Verification items for this drawing (mm, ordinates from the low corner). Give positions to 0.01 mm unless a question says otherwise; leave off trailing zeros. Order: outer loops, then holes, each group sorted by start corner. A loop starts at its lowest first (then second) coordinate and runs counter-clockwise, first axis right, second up. Notation, with made-up numbers: M 67,-14.75 L 82,-14.75 A33 ccw 82,16.25 Z; hole C -9,80.25 d8. An arc over 180 degrees is marked long. Answer as a JSON object with one key per item and string values.
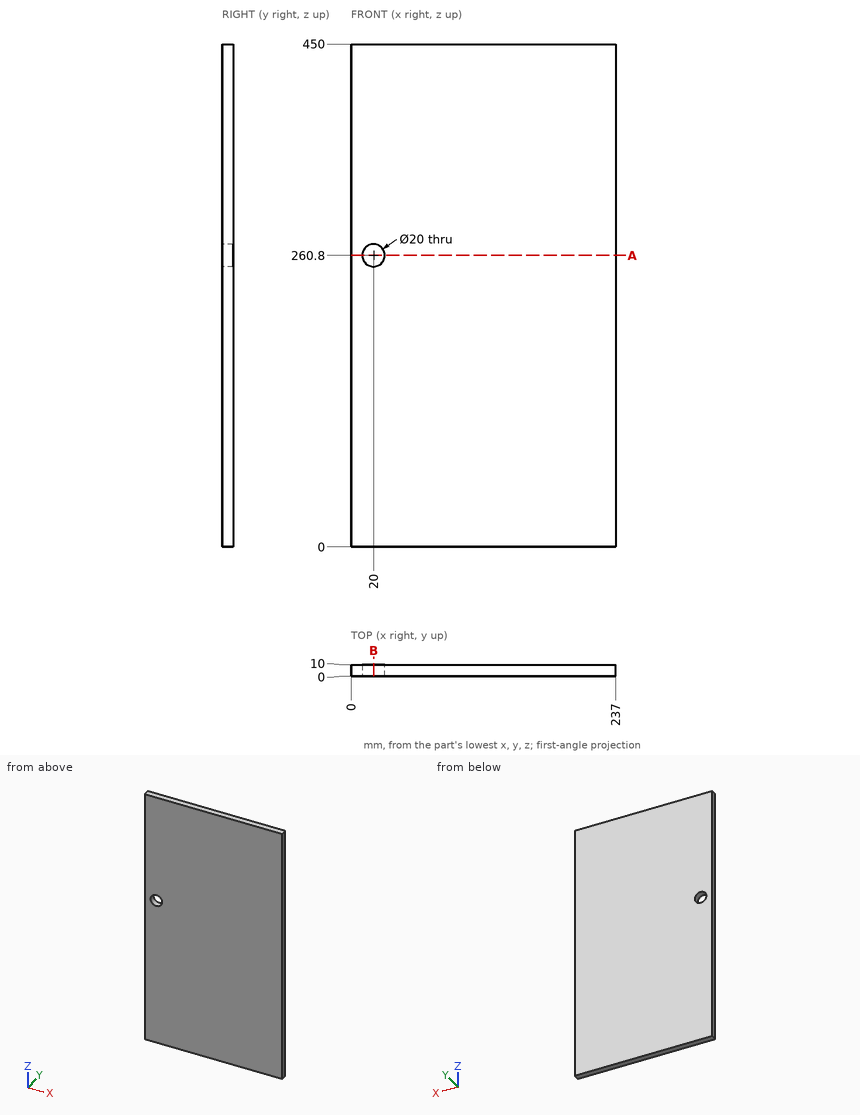
Q1. Material ranges on L1, parallel to Z at x = 20, y = 4.25; L2, parallel to X at y = 8, z = 260.8; L3, parallel to X at y = 8.75, z = 264.5, recorded low to high.
Resolved:
{"L1": "z = 0 to 250.8, 270.8 to 450", "L2": "x = 0 to 10, 30 to 237", "L3": "x = 0 to 10.71, 29.29 to 237"}
Q2. Section check A-A on z = 260.8. Record the cut outline in (x, y).
Resolved:
{"outline": "M 0,0 L 10,0 L 10,10 L 0,10 Z; M 30,0 L 237,0 L 237,10 L 30,10 Z"}
Q3. Section check B-B on x = 20. Record the cut outline in (y, z), then the cut area to 3 significant figures.
Resolved:
{"outline": "M 0,0 L 10,0 L 10,250.8 L 0,250.8 Z; M 0,270.8 L 10,270.8 L 10,450 L 0,450 Z", "area": "4,300 mm²"}
